from build123d import *

# Parameters (mm, degrees)
F0_W     = 38.1
F0_H     = 38.1
F1_DEPTH = 590.55
F2_W     = 38.1
F2_H     = 38.1
F3_DEPTH = 19.05
F4_W     = 38.1
F4_H     = 38.1
F5_DEPTH = 19.05
F6_W     = 38.1
F6_H     = 38.1
F7_DEPTH = 19.05


with BuildPart() as f1:
    # F0 (on Top) → F1 (new body)
    with BuildSketch(Plane.XY):
        with Locations((-34.016462, 22.66462)):
            Rectangle(F0_W, F0_H)
    extrude(amount=F1_DEPTH)

    # F2 (on face) → F3 (cut)
    with BuildSketch(Plane.XZ.offset(-3.61462)):
        with Locations((-34.016462, 571.5)):
            Rectangle(F2_W, F2_H)
    extrude(amount=-F3_DEPTH, mode=Mode.SUBTRACT)

    # F4 (on face) → F5 (cut)
    with BuildSketch(Plane.YZ.offset(-14.966462)):
        with Locations((22.66462, 133.35)):
            Rectangle(F4_W, F4_H)
    extrude(amount=-F5_DEPTH, mode=Mode.SUBTRACT)

    # F6 (on face) → F7 (cut)
    with BuildSketch(Plane.XZ.offset(-3.61462)):
        with Locations((-34.016462, 184.15)):
            Rectangle(F6_W, F6_H)
    extrude(amount=-F7_DEPTH, mode=Mode.SUBTRACT)


solid = f1.part
Build history of the part. All positions in model axes, mm. A direction names the side the tool comes from. Give positions to 0.01 mm unless a question says otherwise; leave off trailing zeros. Order: outer loops, then holes, each group sorted by start corner. A loop starts at its lowest first (then second) coordinate and runs counter-clockwise, first axis right, second up. Notation, with made-up numbers: M -20,84.5 L -6,84.5 A25 cw -6,117.5 Z; hole C 87.25,35.25 d7. An arc over 180 degrees is marked long. Use one line per item in the form item = value.
Q1. Pin check, flat tips, straight feed: P1, Ø1.5, axis at x = -27, y = 21.5, coming from the +Z side; P2, Ø12, axis at x = -44, y = 11.5, coming from the -Z side. Stop position of each tip, or through.
Conclusion:
P1 = 552.45
P2 = 0
Q2. Wall check: probe 1 along Z at (x, y) = (-32, 14); probe 2 along Z at (x, y) = (-51, 22); probe 3 along Z at (x, y) = (-25, 30). Give the ranges that are in metal, low to high.
Conclusion:
probe_1 = 0 to 114.3, 152.4 to 165.1, 203.2 to 552.45
probe_2 = 0 to 165.1, 203.2 to 552.45
probe_3 = 0 to 114.3, 152.4 to 590.55
Q3. Slice it at B-B, the plane x = -21.5. Write the cut outline in (y, z).
Conclusion:
outline = M 3.61,0 L 41.71,0 L 41.71,114.3 L 3.61,114.3 Z; M 3.61,152.4 L 41.71,152.4 L 41.71,590.55 L 22.66,590.55 L 22.66,552.45 L 3.61,552.45 L 3.61,203.2 L 22.66,203.2 L 22.66,165.1 L 3.61,165.1 Z
Q4. Slice it at C-C, the plane x = -47. Write the cut outline in (y, z).
Conclusion:
outline = M 3.61,0 L 41.71,0 L 41.71,590.55 L 22.66,590.55 L 22.66,552.45 L 3.61,552.45 L 3.61,203.2 L 22.66,203.2 L 22.66,165.1 L 3.61,165.1 Z
Q5. Slice it at D-D, the plane y = 36.5. Write the cut outline in (x, z).
Conclusion:
outline = M -53.07,0 L -14.97,0 L -14.97,114.3 L -34.02,114.3 L -34.02,152.4 L -14.97,152.4 L -14.97,590.55 L -53.07,590.55 Z
Q6. Which spindle directions (+Z, -Z, +X, -X, +Y, -Y) get a long thin tool onto all of the face, cutting with end or side? Do faces 1 (the flat face through (-34, 22.665, 572)), 2 (the flat face through (-34, 13, 203.2)), 3 (the flat face through (-53.066, 22, 291)), 4 (the flat face through (-34.016, 22, 134)), 5 (the flat face through (-34, 41.715, 291)). Say none if no direction does.
Conclusion:
face_1 = +Z, +X, -X, -Y
face_2 = +X, -X, -Y
face_3 = +Z, -Z, -X, +Y, -Y
face_4 = +X, +Y, -Y
face_5 = +Z, -Z, +X, -X, +Y
Q7. Slice it at A-A, the plane y = 12. Write the cut outline in (x, z).
Conclusion:
outline = M -53.07,0 L -14.97,0 L -14.97,114.3 L -34.02,114.3 L -34.02,152.4 L -14.97,152.4 L -14.97,165.1 L -53.07,165.1 Z; M -53.07,203.2 L -14.97,203.2 L -14.97,552.45 L -53.07,552.45 Z
Q8. Pull direction Z, two halves, no side cores. Call faces 6 (the flat face through (-34, 23, 0)), 7 (the flat face through (-34, 22.665, 184)), 8 (the flat face through (-34, 13, 552.45)): released by +Z, released by -Z, zero draft, split by the parting line, or undercut.
Conclusion:
face_6 = released by -Z
face_7 = undercut
face_8 = released by +Z
